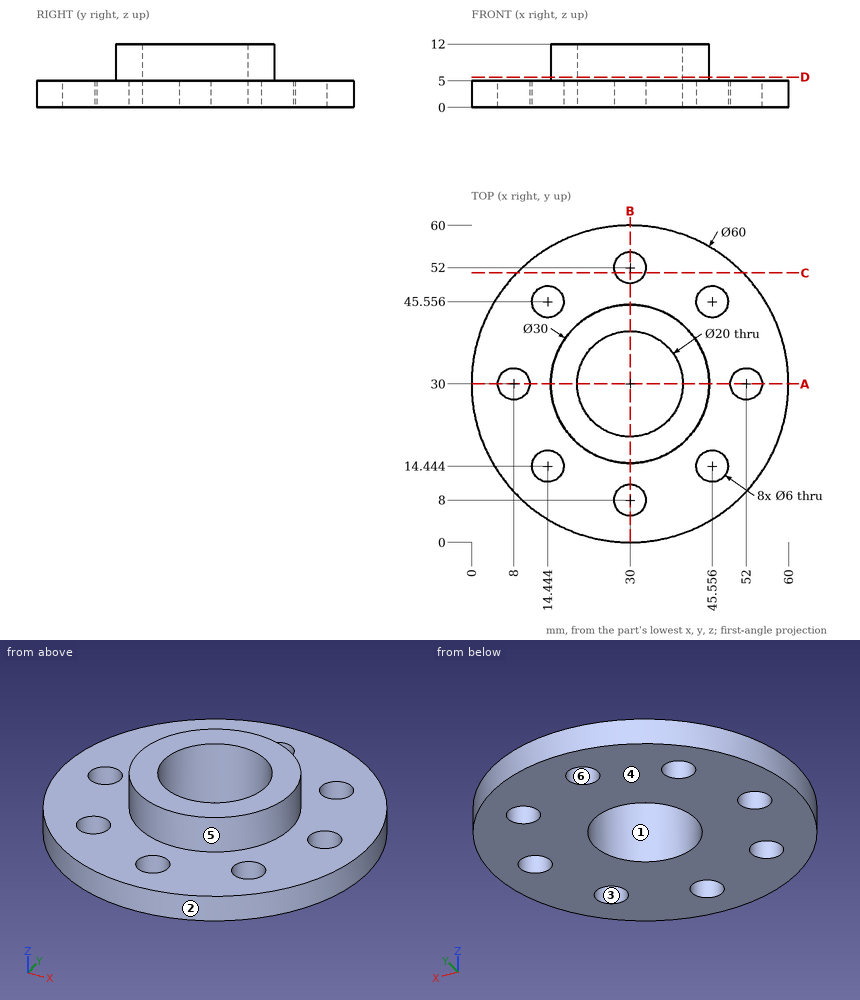
Geometry check sheet. Reference: drawing and pictorial views, mm from the part's lowest x, y, z. A direction names the side the tool comes from. Round coordinates to 2 decimals unless told otherwise and drop trailing zeros. Loops run counter-clockwise (first coordinate to the right, second up) from the corner with the lowest first, then second, coordinate; pieces in that order, holes last. Notation, with made-up numbers: (63, 84) - (122, 84) arc R11 ccw to (122, 92) - close; hole circle Ø9 at (35.25, 65). An arc over 180 degrees is marked (long way). Answer as CSV lines item,"result".
(1) Cross-section at A-A, the plane y = 30. Enter the section's corners in (x, z).
Output values:
outline,"(0, 0) - (5, 0) - (5, 5) - (0, 5) - close; (11, 0) - (20, 0) - (20, 12) - (15, 12) - (15, 5) - (11, 5) - close; (40, 0) - (49, 0) - (49, 5) - (45, 5) - (45, 12) - (40, 12) - close; (55, 0) - (60, 0) - (60, 5) - (55, 5) - close"
(2) Cross-section at D-D, the plane z = 5.75. Enter the section's corners in (x, y).
Output values:
outline,"circle Ø30 at (30, 30); hole circle Ø20 at (30, 30)"
(3) Cross-section at C-C, the plane y = 51. Enter the section's corners in (x, z).
Output values:
outline,"(8.58, 0) - (27.17, 0) - (27.17, 5) - (8.58, 5) - close; (32.83, 0) - (51.42, 0) - (51.42, 5) - (32.83, 5) - close"
(4) Set-up check for the marked faces 5 and 6: record each of +Z, -Z, +X, -X, +Y, -Y from which the full face is reachable in a straight line by a thin tool's end or side.
Output values:
face 5,"+Z"
face 6,"+Z, -Z"
(5) Depth check by flat-ended pin: pin 1 Ø1.5 at (y, z) = (17.5, 3.5) entering from -X; pin 2 Ø5 at (y, z) = (23, 3) entering from -X; pin 3 Ø3 at (x, y) = (44, 51) entering from +Z. Enter the tip coordinate at first touch or a pass-through.
Output values:
pin 1,"stops at x = 2.4"
pin 2,"stops at x = 0.34"
pin 3,"stops at z = 5"
(6) Material ranges on line 1 along X through (y, z) = (30, 7.5); line 2 along Y through (x, z) = (12.5, 4); line 3 along X through (y, z) = (17, 2.75) (1 decimal), recorded low to high.
Output values:
line 1,"x = 15 to 20, 40 to 45"
line 2,"y = 5.63 to 12.16, 16.73 to 43.27, 47.84 to 54.37"
line 3,"x = 3 to 12.9, 16 to 44, 47.1 to 57"
(7) Release check for a two-part mould opening along Y. For the marked faces 1, 2, 3 and 4 record: released by +Y, released by -Y, zero draft, split by the parting line, or undercut.
Output values:
face 1,"undercut"
face 2,"split by the parting line"
face 3,"undercut"
face 4,"zero draft"
